from build123d import *

# Parameters (mm, degrees)
BOSS_EXTRUDE3_DEPTH   = 72.39
BOSS_EXTRUDE5_DEPTH   = 2.5
BOSS_EXTRUDE6_START   = 69.89
BOSS_EXTRUDE6_DEPTH   = 2.5
F_3_0MM_DOWEL_HOLE2_D = 3
F_3_0MM_DOWEL_HOLE3_D = 3


with BuildPart() as part:
    # Sketch1 → Boss-Extrude3 (new body)
    with BuildSketch(Plane(origin=(0, 0, 0), x_dir=(1, 0, 0), z_dir=(0, 1, 0))):
        with BuildLine():
            Line((13.491537447, 0), (17.666973025, 0))
            Line((17.666973025, 0), (17.666973025, -1.92406576))
            Line((17.666973025, -1.92406576), (14.860010366, -1.92406576))
            ThreePointArc((14.860010366, -1.92406576), (-0.00846255, -14.992448629), (-14.876935466, -1.92406576))
            Line((-14.876935466, -1.92406576), (-17.683026975, -1.92406576))
            Line((-17.683026975, -1.92406576), (-17.683026975, 0))
            Line((-17.683026975, 0), (-13.508462552, 0))
            ThreePointArc((-13.508462552, 0), (-0.008462552, -13.5), (13.491537447, 0))
        make_face()
    extrude(amount=BOSS_EXTRUDE3_DEPTH)

    # Sketch8 → Boss-Extrude5 (add)
    with BuildSketch(Plane(origin=(0, 0, 0), x_dir=(1, 0, 0), z_dir=(0, 1, 0))):
        with BuildLine():
            Line((-13.5, 0), (-15, 0))
            ThreePointArc((-15, 0), (0, -15), (15, 0))
            Line((15, 0), (13.5, 0))
            ThreePointArc((13.5, 0), (11.178820599, 7.568617445), (5.013485922, 12.534550607))
            Line((5.013485922, 12.534550607), (5.013485922, -12.534550607))
            ThreePointArc((5.013485922, -12.534550607), (0, -13.5), (-5.013485922, -12.534550607))
            Line((-5.013485922, -12.534550607), (-5.013485922, 12.534550607))
            ThreePointArc((-5.013485922, 12.534550607), (-11.178820599, 7.568617445), (-13.5, 0))
        make_face()
    extrude(amount=BOSS_EXTRUDE5_DEPTH)

    # Sketch8<6> → Boss-Extrude6 (add)
    with BuildSketch(Plane(origin=(0, 0, 0), x_dir=(1, 0, 0), z_dir=(0, 1, 0)).offset(BOSS_EXTRUDE6_START)):
        with BuildLine():
            Line((-13.5, 0), (-15, 0))
            ThreePointArc((-15, 0), (0, -15), (15, 0))
            Line((15, 0), (13.5, 0))
            ThreePointArc((13.5, 0), (11.178820599, 7.568617445), (5.013485922, 12.534550607))
            Line((5.013485922, 12.534550607), (5.013485922, -12.534550607))
            ThreePointArc((5.013485922, -12.534550607), (0, -13.5), (-5.013485922, -12.534550607))
            Line((-5.013485922, -12.534550607), (-5.013485922, 12.534550607))
            ThreePointArc((-5.013485922, 12.534550607), (-11.178820599, 7.568617445), (-13.5, 0))
        make_face()
    extrude(amount=BOSS_EXTRUDE6_DEPTH)

    # Ø3.0mm Dowel Hole2 (through all)
    with Locations(Plane(origin=(0, 0, 0), x_dir=(-1, 0, 0), z_dir=(0, 0, -1))):
        with Locations((15.583026975, 67.54)):
            Hole(F_3_0MM_DOWEL_HOLE2_D / 2)

    # Ø3.0mm Dowel Hole3 (through all)
    with Locations(Plane(origin=(0, 0, 0), x_dir=(-1, 0, 0), z_dir=(0, 0, -1))):
        with Locations((-15.566973025, 67.540028113), (-15.566973025, 4.85), (15.583026975, 4.85)):
            Hole(F_3_0MM_DOWEL_HOLE3_D / 2)


solid = part.part
Work out the finished part from the listing and answer in its coordinate system (mm). A direction names the side the tool comes from. Give positions to 0.01 mm unless a question says otherwise; leave off trailing zeros. Loops run counter-clockwise (first coordinate to the right, second up) from the corner with the lowest first, then second, coordinate; pieces in that order, holes last. Notation, with made-up numbers: (62.5, 67) - (67.5, 67) arc R22 cw to (67.5, 85) - close; hole circle Ø6 at (80.5, 21.5). An arc over 180 degrees is marked (long way). Answer in a Markdown table with one row per item. Add a question column.
Q1. Consider line 1 along Y through (x, z) = (9.5, 5.5); line 2 along X through (y, z) = (4.85, 1.35); line 3 along X through (y, z) = (4.85, 3.35). Determine where each line is inside the solid, lowest interval first.
Q2. Each of these flat-tipped pins is pushed along its axis until it touches: P1, Ø12, axis at x = 14, y = 16, coming from the +Z side; P2, Ø3.5, axis at x = 16.5, y = 21, coming from the -Z side; P3, Ø4, axis at y = 44.5, z = 6, coming from the -X side; P4, Ø7, axis at x = -5, z = -4.5, coming from the -Y side. Where does it stop, or does it pass through?
Q3. The part is cut by section C-C (y = 29). Determine the outline of the cut face in (x, z).
Q4. The part is cut by section A-A (y = 4.85). Determine the outline of the cut face in (x, z), and give its area (3 significant figures).
Q5. Determine the mould class of faces 1 (the cylindrical face through (11.24, 1.23, -7.48)), 2 (the flat face through (-5.3, 72.39, 3.2)), 3 (the cylindrical face through (14.07, 67.61, 1.47)) for opening direction X: released by +X, released by -X, zero draft, split by the parting line, or undercut.
Q6. A tool of negligible diameter and unlimited length cuts with its end or side. For faces 4 (the flat face through (8, 2.5, 0)), 5 (the flat face through (-5.013, 71, 0)), from which of +Z, -Z, +X, -X, +Y, -Y can it reach the whole face along a straight path? Write none if from no direction.
Solution:
| question | item | result |
|---|---|---|
| 1 | line 1 | y = 0 to 2.5, 69.89 to 72.39 |
| 1 | line 2 | x = -17.68 to -17.08, -14.08 to -13.44, 13.42 to 14.07, 17.07 to 17.67 |
| 1 | line 3 | x = -14.08 to -13.09, 13.07 to 14.07 |
| 2 | P1 | stops at z = 12.67 |
| 2 | P2 | stops at z = 0 |
| 2 | P3 | stops at x = -14.46 |
| 2 | P4 | stops at y = 0 |
| 3 | outline | (-17.68, 0) - (-13.51, 0) arc R13.5 cw to (13.49, 0) - (17.67, 0) - (17.67, 1.92) - (14.86, 1.92) arc R14.99 ccw to (-14.88, 1.92) - (-17.68, 1.92) - close |
| 4 | outline | (-17.68, 0) - (-17.08, 0) - (-17.08, 1.92) - (-17.68, 1.92) - close; (-14.08, 0) - (-13.51, 0) arc R13.5 cw to (13.49, 0) - (14.07, 0) - (14.07, 5.16) arc R14.99 ccw to (-14.08, 5.17) - close; (17.07, 0) - (17.67, 0) - (17.67, 1.92) - (17.07, 1.92) - close |
| 4 | area | 62.7 mm² |
| 5 | face 1 | released by +X |
| 5 | face 2 | zero draft |
| 5 | face 3 | undercut |
| 6 | face 4 | -Z |
| 6 | face 5 | -Z, +Y, -Y |
